Read the model definition and answer for the solid it produces. Units are mm, in the model's axes. A direction names the side the tool comes from. Give positions to 0.01 mm unless a question says otherwise; leave off trailing zeros. Loops run counter-clockwise (first coordinate to the right, second up) from the corner with the lowest first, then second, coordinate; pieces in that order, holes last. Notation, with made-up numbers: (62.25, 76) - (68.25, 76) arc R22 cw to (68.25, 91) - close; hole circle Ø11 at (22.25, 87). An arc over 180 degrees is marked (long way). Use a Markdown table: item, result. Add a question column.
Item 1: Which of the six approach directions +Z, -Z, +X, -X, +Y, -Y give full straight-line access (tool end or side, diameter ignored) to faces 4 (the face through (1.75, 1, 5)), 5 (the face through (3.75, 4, 5)), 6 (the face through (9.053, 1, 5))?
Item 2: A cutting plane is placed at D-D (x = 4.25). Determine the outline of the cut face in (y, z).
Item 3: A cutting plane is placed at B-B (z = 5.25). Determine the outline of the cut face in (x, y).
Item 4: Each of these flat-tipped pins is pushed along its axis until it touches: P1, Ø2.5, axis at y = 3.5, z = 7.5, coming from the +X side; P2, Ø1.5, axis at x = 6.5, z = 2.5, coming from the +Y side; P3, Ø1.2, axis at x = 6.5, z = 5.5, coming from the +Y side. Where does it stop, or does it pass through?
Item 5: Consider probe 1 along X at (y, z) = (1.35, 5.5); probe 2 along Z at (x, y) = (6.5, 1.05); probe 3 along X at (y, z) = (1.3, 8). Determine where each line is inside the solid, lowest interval first. Write a range as [from, to].
Item 6: A cutting plane is placed at A-A (y = 1.05). Determine the outline of the cut face in (x, z).
Item 7: A cutting plane is placed at C-C (x = 6.5). Determine the outline of the cut face in (y, z), plus the area to 3 significant figures.
Item 8: For a pull along Z with two mould halves and no side action, classify faces 1 (the face through (2, 2, 11)), 2 (the face through (1, 5, 5)), 3 (the face through (5.763, 0.986, 4.824)) as +Z half, -Z half, draft (parallel to the pull), parting line (faces both ways), or undercut.
from build123d import *

# Parameters (mm, degrees)
CYLINDER_R          = 1
CYLINDER_DEPTH      = 10
CYLINDER_ROLL_ANGLE = -90
EXTRUDE_DEPTH       = 11


with BuildPart() as cylinder:
    # Cylinder → Cylinder (new body)
    with BuildSketch(Plane.XY):
        Circle(CYLINDER_R)
    extrude(amount=CYLINDER_DEPTH)


with BuildPart() as cylinder_1:
    # Cylinder roll: moved
    add(cylinder.part.rotate(Axis((0, 0, 0), (1, 0, 0)), CYLINDER_ROLL_ANGLE))


with BuildPart() as cylinder_2:
    # Cylinder placement: moved
    add(cylinder_1.part.moved(Location((6.5, 0, 5.5))))


with BuildPart() as cut:
    # Sketch → Extrude (new body)
    with BuildSketch(Plane.XY):
        Polygon((-2, 0), (-2, 5), (3.75, 5), (3.75, 2), (9.053131, 2), (9.053131, 0), (1.75, 0), (1.75, 3), (0, 3), (0, 0), align=None)
    extrude(amount=EXTRUDE_DEPTH)

    # Cut: cut Cylinder
    add(cylinder_2.part, mode=Mode.SUBTRACT)


solid = cut.part
Geometry says:
| question | item | result |
|---|---|---|
| 1 | face 4 | +Z, -Z, -Y |
| 1 | face 5 | +Z, -Z, +X, +Y |
| 1 | face 6 | +Z, -Z, +X, +Y, -Y |
| 2 | outline | (0, 0) - (2, 0) - (2, 11) - (0, 11) - close |
| 3 | outline | (-2, 0) - (0, 0) - (0, 3) - (1.75, 3) - (1.75, 0) - (5.53, 0) - (5.53, 2) - (3.75, 2) - (3.75, 5) - (-2, 5) - close; (7.47, 0) - (9.05, 0) - (9.05, 2) - (7.47, 2) - close |
| 4 | P1 | x = 3.75 |
| 4 | P2 | y = 2 |
| 4 | P3 | through |
| 5 | probe 1 | [-2, 0], [1.75, 5.5], [7.5, 9.05] |
| 5 | probe 2 | [0, 4.5], [6.5, 11] |
| 5 | probe 3 | [-2, 0], [1.75, 9.05] |
| 6 | outline | (-2, 0) - (0, 0) - (0, 11) - (-2, 11) - close; (1.75, 0) - (9.05, 0) - (9.05, 11) - (1.75, 11) - close; hole circle Ø2 at (6.5, 5.5) |
| 7 | outline | (0, 0) - (2, 0) - (2, 4.5) - (0, 4.5) - close; (0, 6.5) - (2, 6.5) - (2, 11) - (0, 11) - close |
| 7 | area | 18.0 mm² |
| 8 | face 1 | +Z half |
| 8 | face 2 | draft |
| 8 | face 3 | undercut |
